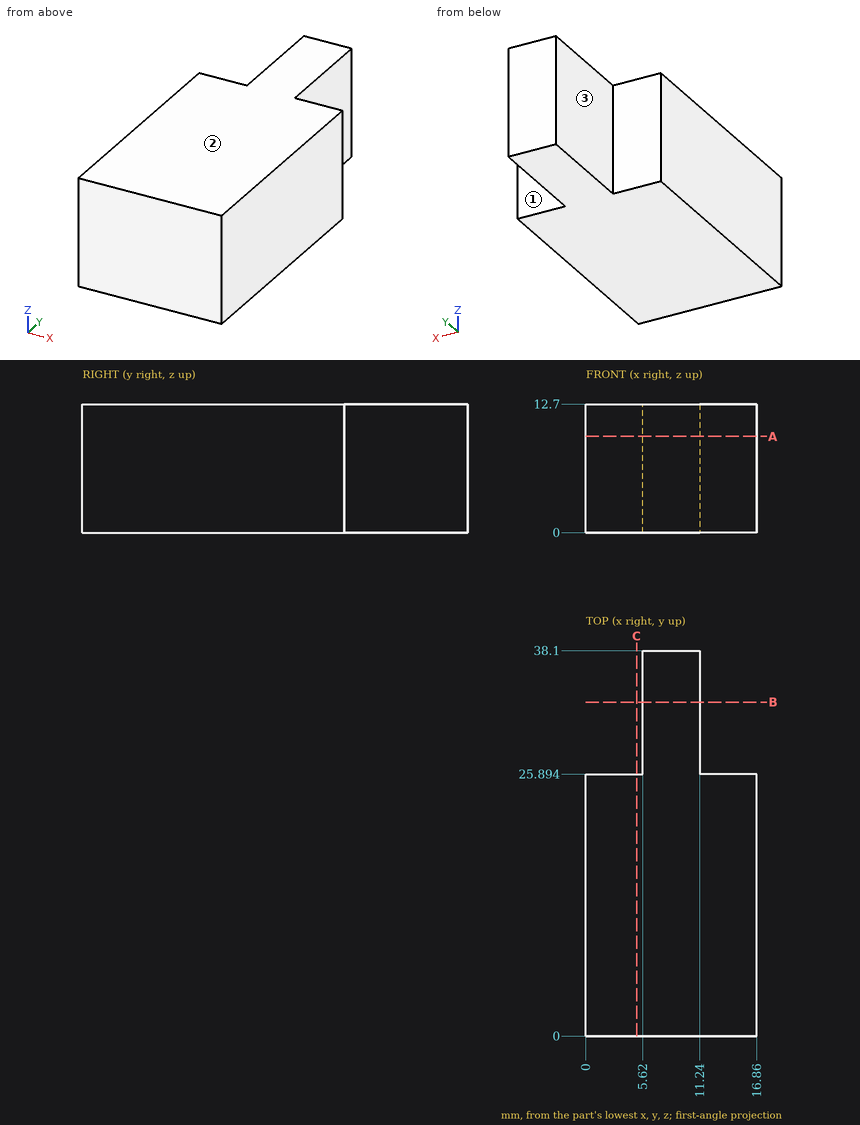
The figure shows three views and two pictorial views of one solid part (mm, origin at its lowest corner). Answer the questions. A direction names the side the tool comes from. Round coordinates to 2 decimals unless told otherwise and drop trailing zeros. Order: outer loops, then holes, each group sorted by start corner. A loop starts at its lowest first (then second) coordinate and runs counter-clockwise, first axis right, second up. Notation, with made-up numbers: M 30.5,-7 L 37.5,-7 A16 ccw 37.5,8 Z; hole C -31,76 d8. An arc over 180 degrees is marked long. Put each result on its own line as item: value. Start each with the question number.
Q1. A tool of negligible diameter and unlimited length cuts with its end or side. For the marked faces 1, 2 and 3, from which of +Z, -Z, +X, -X, +Y, -Y can it reach the whole face along a straight path? Write none if from no direction.
Q2. Flat-ended cylindrical pins translate along their axes: pin 1 (1.7 mm diameter, centred on x = 15, z = 9, fed in from +Y); pin 2 (6 mm diameter, centred on x = 3, y = 32.5, fed in from -Z); pin 3 (3.5 mm diameter, centred on y = 33, z = 6.5, fed in from +X); pin 4 (6 mm diameter, centred on y = 30.5, z = 4.5, fed in from -X). Find the tip coordinate at first contact, or state that the pin passes through.
Q3. Section A-A, the plane z = 9.5 is taken. Write down the section's boundary in (x, y).
Q4. Section B-B, the plane y = 33 is taken. Write down the section's boundary in (x, z).
Q5. Straight lines are drawn through the part: L1, parallel to X at y = 30, z = 8; L2, parallel to Y at x = 15, z = 2. For each, find the intervals that lie inside material, in ascending order. Write a range as [from, to].
Q6. Section C-C, the plane x = 5 is taken. Write down the section's boundary in (y, z), and give its area (3 significant figures).
Findings below:
1. face 1: +Z, -Z, +X, +Y
1. face 2: +Z, +X, -X, +Y, -Y
1. face 3: +Z, -Z, -X, +Y
2. pin 1: stops at y = 25.89
2. pin 2: stops at z = 0
2. pin 3: stops at x = 11.24
2. pin 4: stops at x = 5.62
3. outline: M 0,0 L 16.86,0 L 16.86,25.89 L 11.24,25.89 L 11.24,38.1 L 5.62,38.1 L 5.62,25.89 L 0,25.89 Z
4. outline: M 5.62,0 L 11.24,0 L 11.24,12.7 L 5.62,12.7 Z
5. L1: x = [5.62, 11.24]
5. L2: y = [0, 25.89]
6. outline: M 0,0 L 25.89,0 L 25.89,12.7 L 0,12.7 Z
6. area: 329 mm^2
